Geometry: final body of the model. Coordinates: model frame, mm. Face numbers are marked on the shaded views. A direction names the side the tool comes from. Coordinates: 2 decimals unless noted, no trailing zeros. Write each loop counter-clockwise with the first axis right and the second up, starting at its lowest first coordinate (ties: lowest second). Pieces come first, ordered by that corner, then holes. Notation, with made-up numbers: (6.5, 0.25) - (31.5, 0.25) arc R31 cw to (31.5, 34.25) - close; hole circle Ø3 at (5.5, 30). An arc over 180 degrees is marked (long way). Put each result on its own line as item: value.
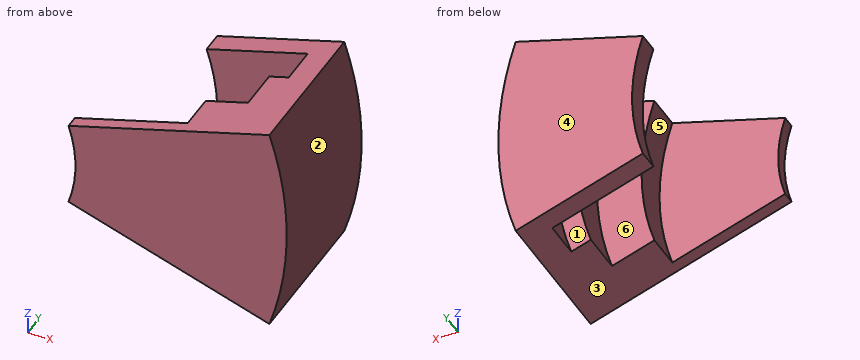
```python
from build123d import *

# Parameters (mm, degrees)
REVOLVE1_ANGLE           = 18
REVOLVE1_OTHER_WAY_ANGLE = 18


with BuildPart() as part:
    # Sketch2 → Revolve1 (revolve)
    with BuildSketch(Plane.XY):
        Polygon((10.35, 112.53957189), (19, 112.53957189), (19, 115.08957189), (22.25, 115.08957189), (22.25, 118.08957189), (23.75, 118.08957189), (23.75, 120.78957189), (16, 120.78957189), (16, 122.28957189), (25.75, 122.28957189), (25.75, 111.63957189), (10.35, 111.63957189), align=None)
    revolve(axis=Axis((0, -1000, 0), (0, 1, 0)), revolution_arc=REVOLVE1_ANGLE)

    # Sketch2 → Revolve1 other way (revolve)
    with BuildSketch(Plane.XY):
        Polygon((10.35, 112.53957189), (19, 112.53957189), (19, 115.08957189), (22.25, 115.08957189), (22.25, 118.08957189), (23.75, 118.08957189), (23.75, 120.78957189), (16, 120.78957189), (16, 122.28957189), (25.75, 122.28957189), (25.75, 111.63957189), (10.35, 111.63957189), align=None)
    revolve(axis=Axis((0, -1000, 0), (0, -1, 0)), revolution_arc=REVOLVE1_OTHER_WAY_ANGLE)


solid = part.part
```
1. Ray query, probe 1 along Y at (x, z) = (16, -2.75); probe 2 along Y at (x, z) = (21.75, -0.5); probe 3 along Y at (x, z) = (13, 1). Return the intervals inside material, ascending. Write a range as from..to.
Answer below:
probe 1: y = 111.64..112.54, 120.79..122.29
probe 2: y = 111.64..115.09, 120.79..122.29
probe 3: y = 111.64..112.54
2. Section query A-A (x = 20.75). Return loops of the section in (y, z), then the cut area to 3 significant figures.
Answer below:
outline: (111.64, -6.74) - (115.09, -6.74) - (115.09, 6.74) - (111.64, 6.74) - close; (120.79, -6.74) - (122.29, -6.74) - (122.29, 6.74) - (120.79, 6.74) - close
area: 66.7 mm²
3. Mould query, pull axis Z, two halves, no side actions, for the marked faces 3, 4, 5 and 6. Classes: +Z half, -Z half, draft (parallel to the pull), parting line (faces both ways), or undercut.
Answer below:
face 3: -Z half
face 4: draft
face 5: undercut
face 6: undercut
4. Section query D-D (z = 1). Return loops of the section in (x, y), then the cut area to 3 significant figures.
Answer below:
outline: (10.3, 111.64) - (25.73, 111.64) - (25.73, 122.29) - (15.97, 122.29) - (15.97, 120.79) - (23.73, 120.79) - (23.73, 118.09) - (22.23, 118.09) - (22.23, 115.09) - (18.97, 115.09) - (18.97, 112.54) - (10.3, 112.54) - close
area: 61.7 mm²
5. Section query C-C (y = 117.5). Return loops of the section in (x, z).
Answer below:
outline: (21.16, -6.88) - (24.49, -7.96) arc R25.75 ccw to (24.49, 7.96) - (21.16, 6.88) arc R22.25 cw to start
6. Set-up query: the marked faces 1 and 2. Return all of +Z, -Z, +X, -X, +Y, -Y with unobstructed straight access to the full face (end or side cutting, diameter ignored); none if empty.
Answer below:
face 1: -X
face 2: +X, +Y, -Y
7. Pin query (flat end, axial travel): pin 1 Ø3 at (y, z) = (118.5, -6) entering from -X; pin 2 Ø5 at (y, z) = (113.5, 0.5) entering from +X; pin 3 Ø1.5 at (y, z) = (118.5, -4.5) entering from -X. Return the tip coordinate at first contact, or that it passes through.
Answer below:
pin 1: stops at x = 21.16
pin 2: stops at x = 25.75
pin 3: stops at x = 21.65
8. Section query B-B (z = -2). Return loops of the section in (x, y), then the cut area to 3 significant figures.
Answer below:
outline: (10.15, 111.64) - (25.67, 111.64) - (25.67, 122.29) - (15.87, 122.29) - (15.87, 120.79) - (23.67, 120.79) - (23.67, 118.09) - (22.16, 118.09) - (22.16, 115.09) - (18.89, 115.09) - (18.89, 112.54) - (10.15, 112.54) - close
area: 61.9 mm²
